```python
from build123d import *

# Parameters (mm, degrees)
SKETCH1_W             = 10.16
SKETCH1_H             = 2.54
BOSS_EXTRUDE1_DEPTH   = 17.526
BOSS_EXTRUDE1_2_DEPTH = 17.526
SKETCH2_W             = 10.16
SKETCH2_H             = 43.434
BOSS_EXTRUDE2_DEPTH   = 2.54
SKETCH3_R             = 1.319522672
SKETCH3_R_2           = 1.34985913
BOSS_EXTRUDE3_DEPTH   = 2.54


with BuildPart() as part:
    # Sketch1 → Boss-Extrude1 (new body)
    with BuildSketch(Plane(origin=(0, 0, 0), x_dir=(1, 0, 0), z_dir=(0, 1, 0))):
        with Locations((-19.169529412, 14.552705882)):
            Rectangle(SKETCH1_W, SKETCH1_H)
    extrude(amount=BOSS_EXTRUDE1_DEPTH)



with BuildPart() as body_2:
    # Sketch1 → Boss-Extrude1 2 (new body)
    with BuildSketch(Plane(origin=(0, 0, 0), x_dir=(1, 0, 0), z_dir=(0, 1, 0))):
        with Locations((-19.169529412, -26.341294118)):
            Rectangle(SKETCH1_W, SKETCH1_H)
    extrude(amount=BOSS_EXTRUDE1_2_DEPTH)


with BuildPart() as part_1:
    add(part.part)

    add(body_2.part)  # Boss-Extrude2 merges body 2
    # Sketch2 → Boss-Extrude2 (add)
    with BuildSketch(Plane(origin=(0, 17.526, 0), x_dir=(1, 0, 0), z_dir=(0, 1, 0))):
        with Locations((-19.169529412, -5.894294118)):
            Rectangle(SKETCH2_W, SKETCH2_H)
    extrude(amount=BOSS_EXTRUDE2_DEPTH)

    # Sketch3 → Boss-Extrude3 (add)
    # profile 1 of 2: a face of its own
    with BuildSketch(Plane.XZ):
        with BuildLine():
            Line((-22.386628374, 27.611294118), (-14.089529412, 27.611294118))
            ThreePointArc((-14.089529412, 27.611294118), (-18.238078893, 31.759843599), (-22.386628374, 27.611294118))
        make_face()
        with Locations(Location((-18.238078893, 29.643294118, 0), (0, 0, 270))):
            Circle(SKETCH3_R, mode=Mode.SUBTRACT)
    # profile 2 of 2: a face of its own
    with BuildSketch(Plane.XZ):
        with BuildLine():
            Line((-22.386628374, -15.822705882), (-14.089529412, -15.822705882))
            ThreePointArc((-14.089529412, -15.822705882), (-18.238078893, -19.971255363), (-22.386628374, -15.822705882))
        make_face()
        with Locations(Location((-18.238078893, -17.854705882, 0), (0, 0, 270))):
            Circle(SKETCH3_R_2, mode=Mode.SUBTRACT)
    extrude(amount=-BOSS_EXTRUDE3_DEPTH)


solid = part_1.part
```
Read the model definition and answer for the solid it produces. Units are mm, in the model's axes. A direction names the side the tool comes from. Coordinates: 2 decimals unless noted, no trailing zeros. Loops run counter-clockwise (first coordinate to the right, second up) from the corner with the lowest first, then second, coordinate; pieces in that order, holes last. Notation, with made-up numbers: (27.25, 63.5) - (57.25, 63.5) arc R31 ccw to (57.25, 96.5) - close; hole circle Ø9 at (61.5, -19). An arc over 180 degrees is marked (long way). Answer in a Markdown table with one row per item.
1. Which of the six approach directions +Z, -Z, +X, -X, +Y, -Y give full straight-line access (tool end or side, diameter ignored) to faces 1 (the face through (-18, 2.54, -16)), 2 (the face through (-19, 9, 25.071)), 3 (the face through (-18.15, 1.25, -19.97)), 4 (the face through (-19, 2.54, 28)), 5 (the face through (-24.25, 18, 4))?
Conclusion:
| item | result |
|---|---|
| face 1 | -Z, +X, -X, +Y |
| face 2 | +X, -X, -Y |
| face 3 | -Z, +Y, -Y |
| face 4 | +Z, +X, -X, +Y |
| face 5 | +Z, -Z, -X, +Y, -Y |
2. Find section A-A, the plane y = 3.25. Write down the section's boundary in (x, z).
Conclusion:
| item | result |
|---|---|
| outline | (-24.25, -15.82) - (-14.09, -15.82) - (-14.09, -13.28) - (-24.25, -13.28) - close; (-24.25, 25.07) - (-14.09, 25.07) - (-14.09, 27.61) - (-24.25, 27.61) - close |
3. Find section B-B, the plane x = -23.25. Write down the section's boundary in (y, z), then the cut area to 3 significant figures.
Conclusion:
| item | result |
|---|---|
| outline | (0, -15.82) - (20.07, -15.82) - (20.07, 27.61) - (0, 27.61) - (0, 25.07) - (17.53, 25.07) - (17.53, -13.28) - (0, -13.28) - close |
| area | 199 mm² |
4. Straight lines are drawn through the part: line 1 (Z direction, x = -22, y = 3); line 2 (Y direction, x = -14.75, z = 28); line 3 (Y direction, x = -19.75, z = 24.5). For each, find the intervals that lie inside material, in ascending order.
Conclusion:
| item | result |
|---|---|
| line 1 | z = -15.82 to -13.28, 25.07 to 27.61 |
| line 2 | y = 0 to 2.54 |
| line 3 | y = 17.53 to 20.07 |
5. Find section C-C, the plane x = -19. Write down the section's boundary in (y, z), then the cut area to 3 significant figures.
Conclusion:
| item | result |
|---|---|
| outline | (0, -19.9) - (2.54, -19.9) - (2.54, -18.97) - (0, -18.97) - close; (0, -16.74) - (2.54, -16.74) - (2.54, -15.82) - (20.07, -15.82) - (20.07, 27.61) - (2.54, 27.61) - (2.54, 28.57) - (0, 28.57) - (0, 25.07) - (17.53, 25.07) - (17.53, -13.28) - (0, -13.28) - close; (0, 30.72) - (2.54, 30.72) - (2.54, 31.69) - (0, 31.69) - close |
| area | 209 mm² |
6. Determine the mould class of faces 6 (the face through (-19, 20.066, 6)), 7 (the face through (-19, 9, -13.283)), 8 (the face through (-19, 10, 27.611)) for opening direction Z: +Z half, -Z half, draft (parallel to the pull), parting line (faces both ways), or undercut.
Conclusion:
| item | result |
|---|---|
| face 6 | draft |
| face 7 | undercut |
| face 8 | +Z half |
7. Find section D-D, the plane z = -4. Write down the section's boundary in (x, y), then the cut area to 3 significant figures.
Conclusion:
| item | result |
|---|---|
| outline | (-24.25, 17.53) - (-14.09, 17.53) - (-14.09, 20.07) - (-24.25, 20.07) - close |
| area | 25.8 mm² |
8. Given pin 1 (3 mm diameter, centred on x = -18.24, z = -17.85, fed in from -Y); pin 2 (1 mm diameter, centred on x = -21, z = -3, fed in from -Y); pin 3 (5 mm diameter, centred on y = 8, z = -10, fed in from +X); pin 4 (3.5 mm diameter, centred on x = -19.5, z = -18, fed in from +Y), each flat-ended and moving along its own axis, determine where each tip first touches the part or whether it passes through.
Conclusion:
| item | result |
|---|---|
| pin 1 | stops at y = 0 |
| pin 2 | stops at y = 17.53 |
| pin 3 | passes through |
| pin 4 | stops at y = 2.54 |
